Autodesk Inventor part; units mm, degrees
ref_plane "YZ Plane" through (0, 0, 0) normal (1, 0, 0) x (0, 1, 0)
ref_plane "XZ Plane" through (0, 0, 0) normal (0, 1, 0) x (-1, 0, 0)
ref_plane "XY Plane" through (0, 0, 0) normal (0, 0, 1) x (1, 0, 0)
sketch "Skizze1" plane through (0, 0, 0) normal (0, 0, 1) x (1, 0, 0)
  circle A0 centre (0, 0) radius 40
  line L0 (0, 100) -> (58.7785, 80.9017)
  line L1 (58.7785, 80.9017) -> (95.1057, 30.9017)
  line L2 (95.1057, 30.9017) -> (95.1057, -30.9017)
  line L3 (95.1057, -30.9017) -> (58.7785, -80.9017)
  line L4 (58.7785, -80.9017) -> (0, -100)
  line L5 (0, -100) -> (-58.7785, -80.9017)
  line L6 (-58.7785, -80.9017) -> (-95.1057, -30.9017)
  line L7 (-95.1057, -30.9017) -> (-95.1057, 30.9017)
  line L8 (-95.1057, 30.9017) -> (-58.7785, 80.9017)
  line L9 (-58.7785, 80.9017) -> (0, 100)
  dimension "d0" = 80
  dimension "d1" = 100
extrude "Extrusion1" add sketch "Skizze1" along normal blind 15
sketch "Skizze3" plane through (0, 0, 0) normal (0, 0, -1) x (-1, 0, 0)
  line L0 (-95.1057, -30.9017) -> (-95.1057, 30.9017)
  line L1 (-58.7785, -80.9017) -> (-95.1057, -30.9017)
  line L2 (0, -100) -> (-58.7785, -80.9017)
  line L3 (58.7785, -80.9017) -> (0, -100)
  line L4 (95.1057, -30.9017) -> (58.7785, -80.9017)
  line L5 (95.1057, 30.9017) -> (95.1057, -30.9017)
  line L6 (58.7785, 80.9017) -> (95.1057, 30.9017)
  line L7 (0, 100) -> (58.7785, 80.9017)
  line L8 (-58.7785, 80.9017) -> (0, 100)
  line L9 (-95.1057, 30.9017) -> (-58.7785, 80.9017)
  circle A0 centre (0, 0) radius 40
extrude "Extrusion2" add sketch "Skizze3" along normal blind 15 contours L0 L9 L8 L7 L6 L5 L4 L3 L2 L1 | A0
sketch "Skizze4" plane through (-58.7785, 80.9017, 15) normal (-0.309, 0.9511, 0) x (0.9511, 0.309, 0)
  line L0 (61.8034, 30) -> (0, 30)
  line L1 (40.9017, 30) -> (40.9017, 25)
  line L2 (40.9017, 25) -> (45.9017, 25)
  line L3 (45.9017, 25) -> (45.9017, 20)
  line L4 (45.9017, 20) -> (15.9017, 20)
  line L5 (15.9017, 20) -> (15.9017, 25)
  line L6 (15.9017, 25) -> (20.9017, 25)
  line L7 (20.9017, 25) -> (20.9017, 30)
  point P0 (30.9017, 15)
  dimension "d6" = 20
  dimension "d7" = 10
  dimension "d8" = 30
  dimension "d9" = 15
  dimension "d10" = 5
  dimension "d11" = 5
extrude "Extrusion3" cut sketch "Skizze4" against normal through all
properties part number "Unterteil"
Check sheet for the modelled part. Datum: model origin and axes. Units: mm. A direction names the side the tool comes from. Coordinates: 2 decimals unless noted, no trailing zeros. Loops run counter-clockwise (first coordinate to the right, second up) from the corner with the lowest first, then second, coordinate; pieces in that order, holes last.
1) Access from +Z, -Z, +X, -X, +Y, -Y to the whole of each face (thin tool, end or side, straight path). Record for faces 1 (the face through (76.69, 56.25, -0.21)), 2 (the face through (-95.106, 0, 0)), 3 (the face through (9.1, 4.36, -12.54)), 4 (the face through (-12, -3, -10)), 5 (the face through (1, 1, 0)).
2) Sectioned sample at B-B (y = 0). Record the boundary of the cut face in (x, z), and give its area (3 significant figures).
3) Material ranges on probe 1 along Y at (x, z) = (0, 6.5); probe 2 along X at (y, z) = (-12.5, 2.25); probe 3 along X at (y, z) = (24.5, -8.5), recorded low to high.
4) Sectioned sample at D-D (x = -32.5). Record the boundary of the cut face in (y, z), and give its area (3 significant figures).
5) Release check for a two-part mould opening along Z. For faces 6 (the face through (11, 5, -10)), 7 (the face through (29.801, -90.317, -0.21)), 8 (the face through (0, 1, -5)), 9 (the face through (41, 1, 15)) record: released by +Z, released by -Z, zero draft, split by the parting line, or undercut.
6) Gauge pin test, flat ends, axial feed: pin 1 (12 mm diameter, centred on x = 29, z = -9, fed in from +Y); pin 2 (2 mm diameter, centred on x = 3, z = -0.5, fed in from +Y); pin 3 (1.5 mm diameter, centred on x = -2, z = -8.5, fed in from +Y). Record the tip position at first contact, or that the pin passes through.
7) Sectioned sample at C-C (y = 21). Record the boundary of the cut face in (x, z), and give its area (3 significant figures).
8) Sectioned sample at A-A (x = 24.5). Record the boundary of the cut face in (y, z), and give its area (3 significant figures).
Check sheet entries:
1. face 1: +Z, -Z, +X, +Y
1. face 2: +Z, -Z, -X, +Y, -Y
1. face 3: -Z
1. face 4: none
1. face 5: +Z
2. outline: (-95.11, -15) - (-10.51, -15) - (-10.51, -10) - (-15.77, -10) - (-15.77, -5) - (15.77, -5) - (15.77, -10) - (10.51, -10) - (10.51, -15) - (95.11, -15) - (95.11, 15) - (40, 15) - (40, 0) - (-40, 0) - (-40, 15) - (-95.11, 15) - close
2. area: 4,240 mm2
3. probe 1: y = -100 to -40, 40 to 100
3. probe 2: x = -95.11 to -38, 38 to 95.11
3. probe 3: x = -95.11 to -23.73, 7.81 to 95.11
4. outline: (-89.44, -15) - (67.66, -15) - (67.66, -10) - (51.48, -10) - (51.48, -5) - (89.44, -5) - (89.44, 15) - (23.32, 15) - (23.32, 0) - (-23.32, 0) - (-23.32, 15) - (-89.44, 15) - close
4. area: 4,370 mm2
5. face 6: undercut
5. face 7: zero draft
5. face 8: undercut
5. face 9: released by +Z
6. pin 1: stops at y = 92.53
6. pin 2: stops at y = 99.35
6. pin 3: stops at y = 99.59
7. outline: (-95.11, -15) - (-17.34, -15) - (-17.34, -10) - (-22.6, -10) - (-22.6, -5) - (8.95, -5) - (8.95, -10) - (3.69, -10) - (3.69, -15) - (95.11, -15) - (95.11, 15) - (34.04, 15) - (34.04, 0) - (-34.04, 0) - (-34.04, 15) - (-95.11, 15) - close
7. area: 4,420 mm2
8. outline: (-92.04, -5) - (-26.86, -5) - (-26.86, -10) - (-43.04, -10) - (-43.04, -15) - (92.04, -15) - (92.04, 15) - (31.62, 15) - (31.62, 0) - (-31.62, 0) - (-31.62, 15) - (-92.04, 15) - close
8. area: 4,000 mm2
